Could you check a few things on this model? Use its own coordinates, in mm. A direction names the side the tool comes from. Coordinates: 2 decimals unless noted, no trailing zeros. Loops run counter-clockwise (first coordinate to the right, second up) from the corner with the lowest first, then second, coordinate; pieces in that order, holes last. Notation, with made-up numbers: (19, 10) - (78, 10) arc R24 ccw to (78, 28) - close; hole circle Ø6 at (-8.5, -38). An arc over 180 degrees is marked (long way). One line per item, written item: value. Start each with the question number.
(1) If we section it at B-B on y = -3: Write out the boundary of the cut face in (x, z), then the cut area to 3 significant figures.
(2) If we mould it in two halves opening along Z, with no side actions, what happens to faces 1 (the face through (-180, 0, 40)), 2 (the face through (-155.868, -6.261, -17.543)), 3 (the face through (-182, -6, 31.929))? For each: pulls with the +Z half, pulls with the -Z half, needs draft (parallel to the pull), parting line crosses it, or undercut.
(3) If we section it at C-C on z = 24: Write out the boundary of the cut face in (x, y).
(4) If we section it at D-D on z = 37.5: Write out the boundary of the cut face in (x, y).
(5) If I drill on line 1 along X through (y, z) = (-2, 50.5); line 2 along Z through (x, y) = (-169, -10); line 3 along Z through (x, y) = (-190, -6.5), over which ranges is the centre line in solid material (lowest first)? Write a range as from..to.
(6) On a 3-axis mill with a long thin cutter (end or side, diameter ignored), from which of +Z, -Z, +X, -X, +Y, -Y can I reach the whole of each face in a straight line? I mean faces 4 (the face through (-159.7, -6.4, 56.5)), 5 (the face through (-180, -12.7, 40)). Say none if no direction works.
(7) If we section it at A-A on z = 10.5: Write out the boundary of the cut face in (x, y), then the cut area to 3 significant figures.
(8) I'm going to push flat-ended pins straight in: P1, Ø6, axis at x = -176, y = -5, coming from the +Z side; P2, Ø6, axis at y = -7.5, z = 7.5, coming from the -X side; P3, Ø2, axis at y = -3.5, z = 5.5, coming from the -X side; P4, Ø10, axis at x = -212.5, z = -11, coming from the +Y side. Where does each tip first touch, or does it pass through?
```python
from build123d import *

# Parameters (mm, degrees)
F0_R     = 51.018803
F1_DEPTH = 12.7
F2_W     = 44.067815
F2_H     = 31.929322
F3_DEPTH = 25.4
F5_DEPTH = 25.4
F6_R     = 7.711808
F7_DEPTH = 25.4


with BuildPart() as f1:
    # F0 (on Front) → F1 (new body)
    with BuildSketch(Plane.XZ):
        with Locations((-179.4101, 27.719645)):
            Circle(F0_R)
    extrude(amount=F1_DEPTH)

    # F2 (on face) → F3 (cut)
    with BuildSketch(Plane.XZ.offset(12.7)):
        with Locations((-181.2303, 15.964661)):
            Rectangle(F2_W, F2_H)
    extrude(amount=-F3_DEPTH, mode=Mode.SUBTRACT)

    # F4 (on face) → F5 (cut)
    with BuildSketch(Plane.XZ.offset(12.7)):
        Polygon((-171.511427, 57.43108), (-171.511427, 47.959364), (-162.50329, 45.032443), (-156.935955, 52.695222), (-162.50329, 60.358001), align=None)
    extrude(amount=-F5_DEPTH, mode=Mode.SUBTRACT)

    # F6 (on face) → F7 (cut)
    with BuildSketch(Plane.XZ.offset(12.7)):
        with Locations((-194.455087, 54.694314)):
            Circle(F6_R)
    extrude(amount=-F7_DEPTH, mode=Mode.SUBTRACT)


solid = f1.part
```
Values:
1. outline: circle Ø102.04 at (-179.41, 27.72); hole (-203.26, 0) - (-159.2, 0) - (-159.2, 31.93) - (-203.26, 31.93) - close; hole circle Ø15.42 at (-194.46, 54.69); hole (-171.51, 47.96) - (-162.5, 45.03) - (-156.94, 52.7) - (-162.5, 60.36) - (-171.51, 57.43) - close
1. area: 6,430 mm2
2. face 1: needs draft
2. face 2: parting line crosses it
2. face 3: undercut
3. outline: (-230.29, -12.7) - (-203.26, -12.7) - (-203.26, 0) - (-230.29, 0) - close; (-159.2, -12.7) - (-128.53, -12.7) - (-128.53, 0) - (-159.2, 0) - close
4. outline: (-229.48, -12.7) - (-129.34, -12.7) - (-129.34, 0) - (-229.48, 0) - close
5. line 1: x = -225.06..-200.93, -187.98..-171.51, -158.53..-133.76
5. line 2: z = -22.23..0, 31.93..47.14, 58.25..77.67
5. line 3: z = -22.19..0, 31.93..48.4, 60.99..77.63
6. face 4: +Y, -Y
6. face 5: +Z, -Z, +X, -X, -Y
7. outline: (-227.44, -12.7) - (-203.26, -12.7) - (-203.26, 0) - (-227.44, 0) - close; (-159.2, -12.7) - (-131.39, -12.7) - (-131.39, 0) - (-159.2, 0) - close
7. area: 660 mm2
8. P1: stops at z = 78.74
8. P2: stops at x = -227.44
8. P3: stops at x = -225.81
8. P4: stops at y = 0
